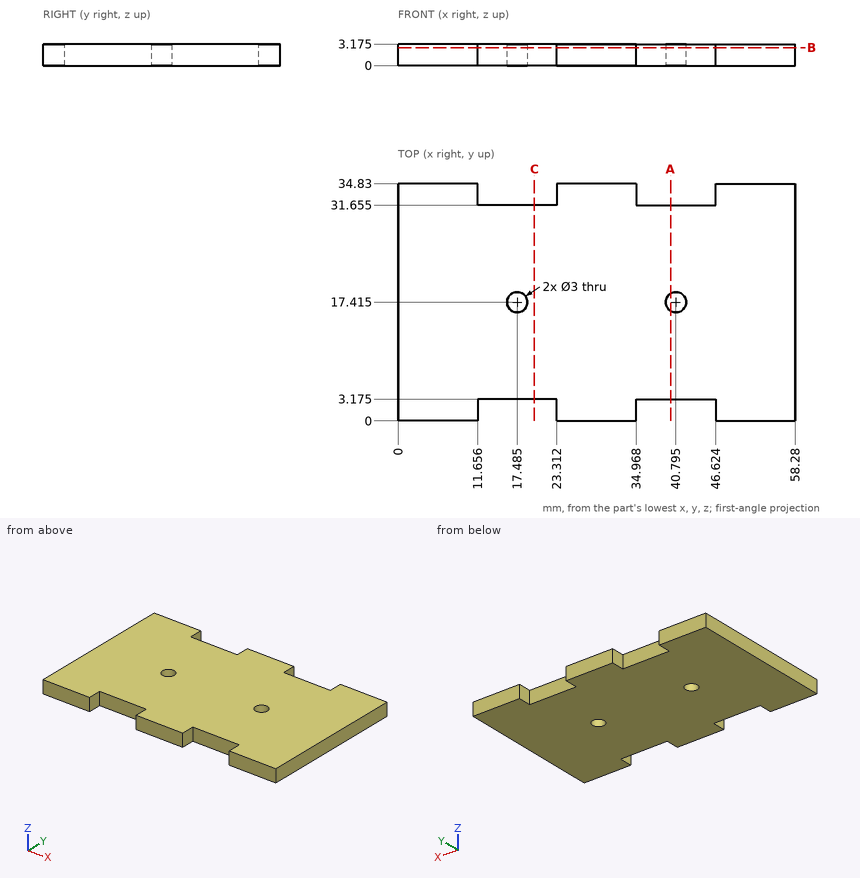
Study the drawing (mm; zero at the part's minimum x, y, z) and answer. Round coordinates to 2 decimals unless told otherwise and drop trailing zeros. Order: outer loops, then holes, each group sorted by start corner. A loop starts at its lowest first (then second) coordinate and runs counter-clockwise, first axis right, second up. Notation, with made-up numbers: (55, 65.25) - (68, 65.25) arc R12 cw to (68, 84.25) - close; hole circle Ø11 at (53, -25.75). An arc over 180 degrees is marked (long way). Use one line per item in the form item = value. Start each with the question number.
(1) The part is cut by section B-B (z = 2.65). Give the vertices of the cut face in (x, y) (3 decimals).
(2) The part is cut by section A-A (x = 40). Give the vertices of the cut face in (y, z) (3 decimals), then the cut area to 3 significant figures.
(3) A flat-ended cylindrical pin translates along its axis: pin 1 Ø5 at (x, y) = (40.795, 17.415) entering from -Z. Find the tip coordinate at first contact, or state that the pin passes through.
(4) The part is cut by section C-C (x = 20). Give the vertices of the cut face in (y, z) (3 decimals), then the cut area to 3 significant figures.
(5) Find the intervals of material crossed by line 1 along Y through (x, z) = (36, 1.7) (3 decimals); line 2 along Y through (x, z) = (42, 0.5) (3 decimals); line 3 along Y through (x, z) = (41.5, 1.45) (3 decimals), in increasing order. Write a range as from..to.
Checked values:
q1.outline = (0, 0) - (11.656, 0) - (11.656, 3.175) - (23.312, 3.175) - (23.312, 0) - (34.968, 0) - (34.968, 3.175) - (46.624, 3.175) - (46.624, 0) - (58.28, 0) - (58.28, 34.83) - (46.624, 34.83) - (46.624, 31.655) - (34.968, 31.655) - (34.968, 34.83) - (23.312, 34.83) - (23.312, 31.655) - (11.656, 31.655) - (11.656, 34.83) - (0, 34.83) - close; hole circle Ø3 at (17.485, 17.415); hole circle Ø3 at (40.795, 17.415)
q2.outline = (3.175, 0) - (16.143, 0) - (16.143, 3.175) - (3.175, 3.175) - close; (18.687, 0) - (31.655, 0) - (31.655, 3.175) - (18.687, 3.175) - close
q2.area = 82.3 mm^2
q3.pin_1 = 0
q4.outline = (3.175, 0) - (31.655, 0) - (31.655, 3.175) - (3.175, 3.175) - close
q4.area = 90.4 mm^2
q5.line_1 = 3.175..31.655
q5.line_2 = 3.175..16.522, 18.308..31.655
q5.line_3 = 3.175..16.091, 18.739..31.655
